Autodesk Inventor part; units mm, degrees
ref_plane "YZ Plane" through (0, 0, 0) normal (1, 0, 0) x (0, 1, 0)
ref_plane "XZ Plane" through (0, 0, 0) normal (0, 1, 0) x (-1, 0, 0)
ref_plane "XY Plane" through (0, 0, 0) normal (0, 0, 1) x (1, 0, 0)
sketch "Sketch1" plane through (0, 0, 0) normal (0, 1, 0) x (-1, 0, 0)
  line L0 (0, 0) -> (-20, 0)
  line L1 (-20, 0) -> (-20, -20)
  line L2 (-20, -20) -> (0, -20)
  line L3 (0, -20) -> (0, 0)
  dimension "d0" = 20
  dimension "d1" = 20
extrude "Extrusion1" add sketch "Sketch1" along normal blind 4
sketch "Sketch2" plane through (0, 4, 0) normal (0, 1, 0) x (1, 0, 0)
  line L0 (0, 0) -> (20, 0)
  line L1 (20, 0) -> (20, 4)
  line L2 (20, 4) -> (4, 4)
  line L3 (0, 4) -> (0, 0)
  line L4 (0, 0) -> (4, 0)
  line L5 (4, 20) -> (0, 20)
  line L6 (0, 20) -> (0, 0)
  line L7 (4, 4) -> (4, 20)
  line L8 (0, 0) -> (20, 0)
  line L9 (0, 0) -> (20, 0)
  line L10 (0, 20) -> (0, 0)
  line L11 (0, 0) -> (0, 20)
extrude "Extrusion2" add sketch "Sketch2" along normal blind 16
hole "Hole2" at (12, 12, -4) direction (0, 0, 1) diameter 4 end through all
hole "Hole3" at (4, 12, -12) direction (-1, 0, 0) diameter 4 end through all
hole "Hole4" at (12, 4, -12) direction (0, -1, 0) diameter 4 end through all
sketch "Sketch3" plane through (20, 4, -4) normal (0, 0, -1) x (-1, 0, 0)
  line L0 (12.0415, 8) -> (10.0207, 4.5)
  line L1 (10.0207, 4.5) -> (5.9793, 4.5)
  line L2 (5.9793, 4.5) -> (3.9585, 8)
  line L3 (3.9585, 8) -> (5.9793, 11.5)
  line L4 (5.9793, 11.5) -> (10.0207, 11.5)
  line L5 (10.0207, 11.5) -> (12.0415, 8)
  point P0 (20, -4)
  point P1 (8, 8)
  dimension "d51" = 7
sketch "Sketch4" plane through (4, 4, -4) normal (1, 0, 0) x (0, 0, -1)
  line L0 (12.0415, 8) -> (10.0207, 4.5)
  line L1 (10.0207, 4.5) -> (5.9793, 4.5)
  line L2 (5.9793, 4.5) -> (3.9585, 8)
  line L3 (3.9585, 8) -> (5.9793, 11.5)
  line L4 (5.9793, 11.5) -> (10.0207, 11.5)
  line L5 (10.0207, 11.5) -> (12.0415, 8)
  point P0 (-4, -4)
  point P1 (8, 8)
  dimension "d52" = 7
sketch "Sketch5" plane through (0, 4, 0) normal (0, 1, 0) x (1, 0, 0)
  circle A0 centre (12, 12) radius 2
  line L0 (12, 7.9585) -> (8.5, 9.9793)
  line L1 (8.5, 9.9793) -> (8.5, 14.0207)
  line L2 (8.5, 14.0207) -> (12, 16.0415)
  line L3 (12, 16.0415) -> (15.5, 14.0207)
  line L4 (15.5, 14.0207) -> (15.5, 9.9793)
  line L5 (15.5, 9.9793) -> (12, 7.9585)
  point P0 (0, 0)
  dimension "d53" = 7
extrude "Extrusion3" cut sketch "Sketch3" against normal blind 2
extrude "Extrusion4" cut sketch "Sketch4" against normal blind 2
extrude "Extrusion5" cut sketch "Sketch5" against normal blind 2
sketch "Sketch6" plane through (0, 0, 0) normal (0, 0, 1) x (1, 0, 0)
  circle A0 centre (25, 25) radius 12
  point P0 (0, 0)
  point P1 (7, 25)
  dimension "d92" = 24
thicken "Thicken3" operation add thickness 18 both sides no extend neighbours yes toward (0, 1, 0) faces at (1.3333, 20, -8)
thicken "Thicken4" operation add thickness 18 both sides no extend neighbours yes toward (1, 0, 0) faces at (20, 14, -1.3333)
hole "Hole5" at (7, 25, 0) direction (0, 0, -1) diameter 8 end through all
extrude "Extrusion6" add sketch "Sketch6" against normal blind 10
hole "Hole7" at (25, 25, 0) direction (0, 0, -1) diameter 10 end through all counterbore diameter 22 counterbore depth 8
properties part number "Frame3WayBlockMotor" material "PLA Orange"
Verification items for the finished model (mm, model axes). A direction names the side the tool comes from. Give positions to 0.01 mm unless a question says otherwise; leave off trailing zeros. Order: outer loops, then holes, each group sorted by start corner. A loop starts at its lowest first (then second) coordinate and runs counter-clockwise, first axis right, second up. Notation, with made-up numbers: (-20, 24.5) -> (26, 24.5) arc R15 cw to (26, 30.5) -> close; hole circle Ø7 at (30.5, 53). An arc over 180 degrees is marked (long way). Use a Markdown table: item, result.
1) Section check D-D, the plane y = 25. Record the boundary of the cut face in (x, z), then the cut area to 3 significant figures.
Results:
| item | result |
|---|---|
| outline | (0, -20) -> (3, -20) -> (3, 0) -> (0, 0) -> close; (11, -4) -> (13, -4) -> (13, -10) -> (20, -10) -> (20, -8) -> (14, -8) -> (14, 0) -> (11, 0) -> close; (30, -10) -> (37, -10) -> (37, -4) -> (38, -4) -> (38, 0) -> (36, 0) -> (36, -8) -> (30, -8) -> close |
| area | 116 mm² |
2) Material ranges on probe 1 along X at (y, z) = (12, -1.1); probe 2 along Y at (x, z) = (25, -5), recorded low to high.
Results:
| item | result |
|---|---|
| probe 1 | 0 to 10, 14 to 38 |
| probe 2 | 0 to 4, 13 to 14, 36 to 37 |
3) Tool access check on faces 1 (the flat face through (3, 10.2, -9)), 2 (the flat face through (3.014, 13.726, -8.955)), 3 (the flat face through (4, 13, -8)), 4 (the flat face through (21, 4, -12)), 5 (the flat face through (21, 13, -4)). Record the directions out of +Z, -Z, +X, -X, +Y, -Y that give a thin tool (end or side, any length) a straight path to the whole face; none if there is none.
Results:
| item | result |
|---|---|
| face 1 | +X |
| face 2 | none |
| face 3 | -Z, +Y |
| face 4 | -Z, +X |
| face 5 | -Z |
4) Section check C-C, the plane z = -3. Record the boundary of the cut face in (x, y).
Results:
| item | result |
|---|---|
| outline | (0, 0) -> (38, 0) -> (38, 38) -> (0, 38) -> close; hole circle Ø8 at (7, 25); hole (7.96, 12) -> (9.98, 8.5) -> (14.02, 8.5) -> (16.04, 12) -> (14.02, 15.5) -> (9.98, 15.5) -> close; hole circle Ø22 at (25, 25) |
5) Mould release check, pull along X, two halves, no side actions. Record for faces 6 (the flat face through (8.5, 3, -12)), 7 (the flat face through (13, 3, -20)): pulls with the +X half, pulls with the -X half, needs draft (parallel to the pull), parting line crosses it, or undercut.
Results:
| item | result |
|---|---|
| face 6 | undercut |
| face 7 | needs draft |
6) Section check A-A, the plane x = 25. Record the boundary of the cut face in (y, z).
Results:
| item | result |
|---|---|
| outline | (0, -20) -> (4, -20) -> (4, -4) -> (13, -4) -> (13, -10) -> (20, -10) -> (20, -8) -> (14, -8) -> (14, 0) -> (0, 0) -> close; (30, -10) -> (37, -10) -> (37, -4) -> (38, -4) -> (38, 0) -> (36, 0) -> (36, -8) -> (30, -8) -> close |
7) Section check B-B, the plane z = -12. Record the boundary of the cut face in (x, y).
Results:
| item | result |
|---|---|
| outline | (0, 0) -> (10, 0) -> (10, 2) -> (8.5, 2) -> (8.5, 4) -> (4, 4) -> (4, 8.5) -> (2, 8.5) -> (2, 10) -> (0, 10) -> close; (0, 14) -> (2, 14) -> (2, 15.5) -> (4, 15.5) -> (4, 22.35) arc R4 cw to (4, 27.65) -> (4, 38) -> (0, 38) -> close; (14, 0) -> (38, 0) -> (38, 4) -> (15.5, 4) -> (15.5, 2) -> (14, 2) -> close |
8) Depth check by flat-ended pin: pin 1 Ø6 at (y, z) = (12, -8) entering from +X; pin 2 Ø6 at (x, y) = (13, 10.5) entering from -Z; pin 3 Ø7.5 at (x, z) = (13.5, -13) entering from +Y. Enter the tip coordinate at first touch or a pass-through.
Results:
| item | result |
|---|---|
| pin 1 | x = 31.63 |
| pin 2 | z = -4 |
| pin 3 | y = 32.64 |
